```python
from build123d import *

# Parameters (mm, degrees)
BOSS_EXTRUDE1_DEPTH = 10


with BuildPart() as part:
    # Sketch1 → Boss-Extrude1 (new body)
    with BuildSketch(Plane(origin=(0, 0, 0), x_dir=(1, 0, 0), z_dir=(0, 1, 0))):
        Polygon((0, 0), (16, 40), (24, 40), (40, 0), (32, 0), (27.2, 12), (12.8, 12), (8, 0), align=None)
        Polygon((16.110598883, 20), (19.781948191, 29.17837327), (23.453297499, 20), align=None, mode=Mode.SUBTRACT)
    extrude(amount=BOSS_EXTRUDE1_DEPTH)


solid = part.part
```
Source: CAD feature listing. Evaluate the final solid. Frame: model axes, mm. A direction names the side the tool comes from. Coordinates: 2 decimals unless noted, no trailing zeros. Write each loop counter-clockwise with the first axis right and the second up, starting at its lowest first coordinate (ties: lowest second). Pieces come first, ordered by that corner, then holes. Notation, with made-up numbers: (-11, 58) -> (-4, 58) arc R23 ccw to (-4, 71) -> close; hole circle Ø8 at (20.25, 69). An arc over 180 degrees is marked (long way). Return JSON: item names as keys, results as strings. Group by question number.
1) Contact query for flat-ended pins moving along their axis: P1, Ø2, axis at y = 1, z = -4.5, coming from the +X side; P2, Ø1, axis at x = 7.5, y = 6.5, coming from the +Z side; P3, Ø3, axis at x = 17.5, y = 5, coming from the +Z side. Output: stop coordinate, or through.
2) Section query C-C, the plane x = 14. Return loops of the section in (y, z), plus the area to 3 significant figures.
3) Section query B-B, the plane y = 5. Return loops of the section in (x, z), plus the area to 3 significant figures.
4) Set-up query: faces 1 (the face through (17.92, 4.93, -24.52)), 2 (the face through (8, 5, -20)), 3 (the face through (20, 5, -12)). Return all of +Z, -Z, +X, -X, +Y, -Y with unobstructed straight access to the full face (end or side cutting, diameter ignored); none if empty.
5) Mould query, pull axis Z, two halves, no side actions, for faces 4 (the face through (20, 0, -16)), 5 (the face through (36, 5, 0)), 6 (the face through (20, 5, -20)), 7 (the face through (20, 5, -40)). Classes: +Z half, -Z half, draft (parallel to the pull), parting line (faces both ways), or undercut.
6) Ray query, line 1 along X through (y, z) = (2.75, -32); line 2 along Z through (x, y) = (23.5, 3.5); line 3 along X through (y, z) = (0.75, -5.5). Return the intervals inside material, ascending.
7) Section query D-D, the plane z = -18. Return loops of the section in (x, y), plus the area to 3 significant figures.
8) Section query A-A, the plane z = -5.5. Return loops of the section in (x, y), plus the area to 3 significant figures.
From the geometry:
{
 "1": {"P1": "x = 38.6", "P2": "z = 0", "P3": "z = -12"},
 "2": {"outline": "(0, -35) -> (10, -35) -> (10, -12) -> (0, -12) -> close", "area": "230 mm²"},
 "3": {"outline": "(0, 0) -> (16, -40) -> (24, -40) -> (40, 0) -> (32, 0) -> (27.2, -12) -> (12.8, -12) -> (8, 0) -> close; hole (16.11, -20) -> (19.78, -29.18) -> (23.45, -20) -> close", "area": "696 mm²"},
 "4": {"face 1": "+Y, -Y", "face 2": "-Z, -X, +Y, -Y", "face 3": "+Z, +Y, -Y"},
 "5": {"face 4": "draft", "face 5": "+Z half", "face 6": "undercut", "face 7": "-Z half"},
 "6": {"line 1": "12.8 to 27.2", "line 2": "-40 to -12", "line 3": "2.2 to 10.2, 29.8 to 37.8"},
 "7": {"outline": "(7.2, 0) -> (32.8, 0) -> (32.8, 10) -> (7.2, 10) -> close", "area": "256 mm²"},
 "8": {"outline": "(2.2, 0) -> (10.2, 0) -> (10.2, 10) -> (2.2, 10) -> close; (29.8, 0) -> (37.8, 0) -> (37.8, 10) -> (29.8, 10) -> close", "area": "160 mm²"}
}
